Design review of the part shown in the three views and the two pictorial views. Dimensions are in mm from the part's minimum x, y and z. A direction names the side the tool comes from. Coordinates: 2 decimals unless noted, no trailing zeros. Loops run counter-clockwise (first coordinate to the right, second up) from the corner with the lowest first, then second, coordinate; pieces in that order, holes last. Notation, with made-up numbers: (8.25, 50.5) -> (59.25, 50.5) arc R8 ccw to (59.25, 65.5) -> close; hole circle Ø4 at (40, 65). An arc over 180 degrees is marked (long way). Use a Markdown table: item, result. Add a question column.
Q1. Clearance check with flat-ended pins moving along their axes: pin 1 Ø3 at (y, z) = (16, 6.5) entering from +X; pin 2 Ø5 at (y, z) = (15, 5) entering from -X; pin 3 Ø4 at (x, y) = (100, 13) entering from -Z; pin 4 Ø2 at (x, z) = (39.5, 10) entering from -Y. State where each tip first meets the part, or that it passes through.
Q2. For probe 1 along Y at (x, z) = (60, 3); probe 2 along X at (y, z) = (10.25, 9.75); probe 3 along Y at (x, z) = (9, 1.25), list the stretches that pass through material, from the lowest coordinate up.
Q3. Take a section at C-C on z = 13.5. Write out the cut boundary in (x, y).
Q4. For the marked faces 5, 6 and 7, list the 3-axis set-ups (+Z, -Z, +X, -X, +Y, -Y) from which the entire face can be reached by the end or side of a thin tool; tool diameter is ignored.
Q5. Draft analysis for pull direction Y (two halves, no side actions). For the marked faces 1, 2, 3 and 4, state which applies: pulls with the +Y half, pulls with the -Y half, needs draft (parallel to the pull), parting line crosses it, or undercut.
Q6. Take a section at A-A on z = 6.5. Write out the cut boundary in (x, y).
Q7. Take a section at B-B on x = 80. Write out the cut boundary in (y, z).
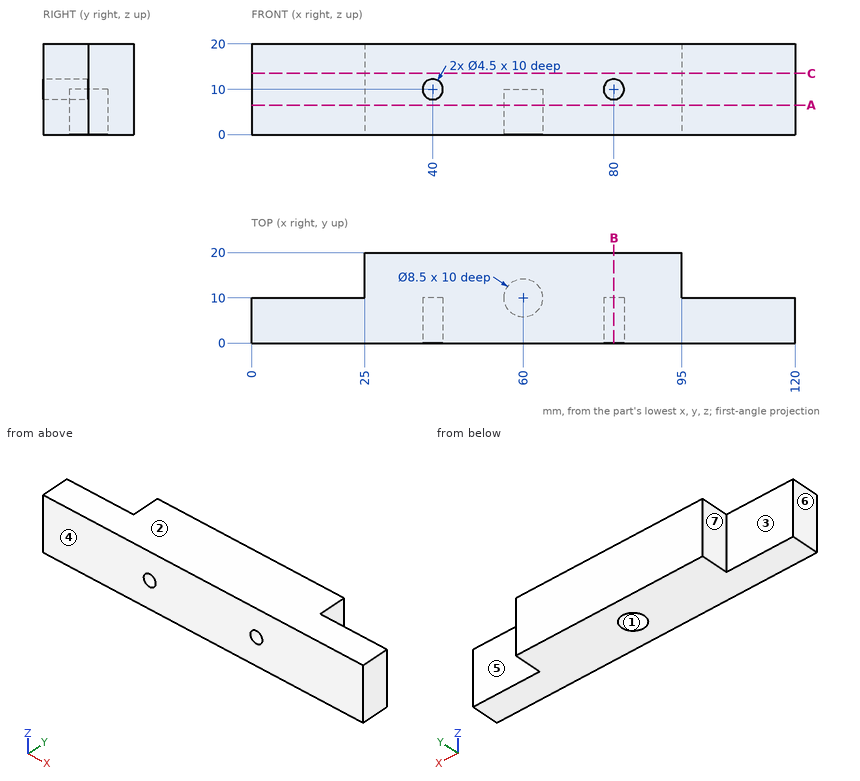
Answer list:
| question | item | result |
|---|---|---|
| 1 | pin 1 | x = 95 |
| 1 | pin 2 | x = 25 |
| 1 | pin 3 | through |
| 1 | pin 4 | y = 10 |
| 2 | probe 1 | 0 to 5.75, 14.25 to 20 |
| 2 | probe 2 | 25 to 55.76, 64.24 to 95 |
| 2 | probe 3 | 0 to 10 |
| 3 | outline | (0, 0) -> (120, 0) -> (120, 10) -> (95, 10) -> (95, 20) -> (25, 20) -> (25, 10) -> (0, 10) -> close |
| 4 | face 5 | +Z, -Z, +X, +Y |
| 4 | face 6 | +Z, -Z, -X, +Y, -Y |
| 4 | face 7 | +Z, -Z, -X, +Y |
| 5 | face 1 | undercut |
| 5 | face 2 | needs draft |
| 5 | face 3 | pulls with the +Y half |
| 5 | face 4 | pulls with the -Y half |
| 6 | outline | (0, 0) -> (120, 0) -> (120, 10) -> (95, 10) -> (95, 20) -> (25, 20) -> (25, 10) -> (0, 10) -> close; hole circle Ø8.5 at (60, 10) |
| 7 | outline | (0, 0) -> (20, 0) -> (20, 20) -> (0, 20) -> (0, 12.25) -> (10, 12.25) -> (10, 7.75) -> (0, 7.75) -> close |
